Autodesk Inventor part; units mm, degrees
ref_plane "YZ Plane" through (0, 0, 0) normal (1, 0, 0) x (0, 1, 0)
ref_plane "XZ Plane" through (0, 0, 0) normal (0, 1, 0) x (-1, 0, 0)
ref_plane "XY Plane" through (0, 0, 0) normal (0, 0, 1) x (1, 0, 0)
sketch "Sketch1" plane through (0, 0, 0) normal (0, 1, 0) x (-1, 0, 0)
  line L0 (450, 0) -> (-450, 0)
  line L1 (-450, 0) -> (-450, 600)
  line L2 (-450, 600) -> (450, 600)
  line L3 (450, 600) -> (450, 0)
  point P0 (0, 0)
  point P1 (0, 0)
  dimension "d0" = 900
  dimension "d1" = 600
extrude "Extrusion1" add sketch "Sketch1" along normal blind 850
sketch "Sketch2" plane through (0, 850, 0) normal (0, 1, 0) x (1, 0, 0)
  line L0 (-325, -500) -> (325, -500)
  line L1 (325, -500) -> (325, -100)
  line L2 (325, -100) -> (-325, -100)
  line L3 (-325, -100) -> (-325, -500)
  line L4 (-325, -500) -> (325, -100) construction
  line L5 (325, -500) -> (-325, -100) construction
  line L6 (-450, 0) -> (-450, -600)
  line L7 (-450, -600) -> (450, -600)
  point P0 (0, 0)
  point P1 (0, -300)
  point P2 (-450, -300)
  point P3 (-450, -300)
  point P4 (0, -600)
  dimension "d4" = 650
  dimension "d5" = 400
extrude "Extrusion2" cut sketch "Sketch2" against normal blind 180
fillet "Fillet1" radius 20 8 edges at (-325, 760, 100) (-325, 670, 300) (0, 670, 100) (-325, 760, 500) (0, 670, 500) (325, 670, 300) (325, 760, 500) (325, 760, 100)
sketch "Sketch3" plane through (-450, 0, 600) normal (0, 0, 1) x (1, 0, 0)
  line L0 (0, 0) -> (900, 0)
  line L1 (900, 0) -> (900, 850)
  line L2 (0, 0) -> (900, 0)
  line L3 (900, 0) -> (900, 120)
  line L4 (900, 120) -> (0, 120)
  line L5 (0, 120) -> (0, 0)
  point P0 (450, 0)
  dimension "d9" = 120
extrude "Extrusion3" cut sketch "Sketch3" against normal blind 20
sketch "Sketch4" plane through (0, 0, 0) normal (1, 0, 0) x (0, 1, 0)
  line L0 (850, 50) -> (1020, 50)
  arc A0 (1020, 50) -> (1050, 80) centre (1020, 80) ccw
  line L1 (1050, 80) -> (1050, 220)
  arc A1 (1050, 220) -> (1020, 250) centre (1020, 220) ccw
  line L2 (1020, 250) -> (990, 250)
  line L3 (850, 600) -> (850, 0)
  line L4 (850, 0) -> (850, 600)
  line L5 (850, 120) -> (850, 100)
  line L6 (850, 120) -> (850, 480)
  line L7 (850, 500) -> (850, 480)
  line L8 (850, 480) -> (850, 500)
  line L9 (850, 480) -> (850, 120)
  line L10 (850, 100) -> (850, 120)
  point P0 (0, 0)
  dimension "d12" = 60
  dimension "d13" = 200
  dimension "d14" = 50
  dimension "d16" = 30
sketch "Sketch5" plane through (0, 850, 0) normal (0, 1, 0) x (1, 0, 0)
  circle A0 centre (0, -50) radius 15
  point P0 (0, 0)
  dimension "d17" = 30
sweep "Sweep1" add profiles "Sketch5" path "Sketch4" path curves L0 A0 L1 A1 L2
properties part number "Mobile lavandino"
Build history of the part. All positions in model axes, mm. A direction names the side the tool comes from. Round coordinates to 2 decimals unless told otherwise and drop trailing zeros. Loops run counter-clockwise (first coordinate to the right, second up) from the corner with the lowest first, then second, coordinate; pieces in that order, holes last.
Item 1: Pin check, flat tip, straight feed: P1, Ø10, axis at x = -53.5, z = 594, coming from the -Y side. Stop position of the tip, or through.
Item 2: Drill centre lines: line 1 along X through (y, z) = (735, 303); line 2 along Y through (x, z) = (-315, 48.5); line 3 along Z through (x, y) = (63, 87.5). Where is each one in solid material? Low to high.
Item 3: Saw through at C-C (z = 316). List the corners of the cut face in (x, y).
Item 4: Saw through at B-B (x = -61). List the corners of the cut face in (y, z), then the cut area to 3 significant figures.
Item 5: Two-plate mould, pull along X, no slides. Class faces 1 (the face through (6, 0, 294)), 2 (the face through (4, 771, 100)), 3 (the face through (450, 419, 296)), 4 (the face through (325, 771, 303)): released by +X, released by -X, zero draft, split by the parting line, or undercut.
Item 6: Saw through at D-D (y = 107.5). List the corners of the cut face in (x, z).
Item 7: Saw through at A-A (z = 133). List the corners of the cut face in (x, y), then the cut area to 3 significant figures.
Item 8: Which spindle directions (+Z, -Z, +X, -X, +Y, -Y) get a long thin tool onto all of the face, cutting with end or side? Do faces 5 (the face through (0, 990, 250)), 6 (the face through (-325, 771, 297)), 7 (the face through (-6, 61, 580)). Say none if no direction does.
Worked answers:
1. P1: stops at y = 120
2. line 1: x = -450 to -325, 325 to 450
2. line 2: y = 0 to 850
2. line 3: z = 0 to 580
3. outline: (-450, 0) - (450, 0) - (450, 850) - (325, 850) - (325, 690) arc R20 cw to (305, 670) - (-305, 670) arc R20 cw to (-325, 690) - (-325, 850) - (-450, 850) - close
4. outline: (0, 0) - (850, 0) - (850, 100) - (690, 100) arc R20 cw to (670, 120) - (670, 480) arc R20 cw to (690, 500) - (850, 500) - (850, 600) - (120, 600) - (120, 580) - (0, 580) - close
4. area: 436,000 mm2
5. face 1: zero draft
5. face 2: undercut
5. face 3: released by +X
5. face 4: undercut
6. outline: (-450, 0) - (450, 0) - (450, 580) - (-450, 580) - close
7. outline: (-450, 0) - (450, 0) - (450, 850) - (325, 850) - (325, 690) arc R20 cw to (305, 670) - (-305, 670) arc R20 cw to (-325, 690) - (-325, 850) - (-450, 850) - close; circle Ø30 at (0, 1050)
7. area: 649,000 mm2
8. face 5: +Z, +X, -X
8. face 6: +Y
8. face 7: +Z, +X, -X, -Y
